from build123d import *

# Parameters (mm, degrees)
BOSS_EXTRUDE1_DEPTH = 10.7
BOSS_EXTRUDE2_DEPTH = 2
CUT_EXTRUDE2_DEPTH  = 17.842989329
CHAMFER1_SIZE       = 0.4


with BuildPart() as part:
    # Sketch1 → Boss-Extrude1 (new body)
    with BuildSketch(Plane.XY):
        Polygon((0, -6.142777017), (2.175697935, -3.768419365), (5.319800946, -3.071388508), (4.351395869, 0), (5.319800946, 3.071388508), (2.175697935, 3.768419365), (0, 6.142777017), (-2.175697935, 3.768419365), (-5.319800946, 3.071388508), (-4.351395869, 0), (-5.319800946, -3.071388508), (-2.175697935, -3.768419365), align=None)
    extrude(amount=-BOSS_EXTRUDE1_DEPTH)

    # Sketch2 → Boss-Extrude2 (add)
    # profile 1 of 2: a face of its own
    with BuildSketch(Plane.XY):
        Polygon((5.924189557, 0), (7.242620565, 4.181528933), (2.962094779, 5.130498653), (0, 8.363057866), (-2.962094779, 5.130498653), (-7.242620565, 4.181528933), (-5.924189557, 0), (-7.242620565, -4.181528933), (-2.962094779, -5.130498653), (0, -8.363057866), (2.962094779, -5.130498653), (7.242620565, -4.181528933), align=None)
        Polygon((5.319800946, -3.071388508), (4.351395869, 0), (5.319800946, 3.071388508), (2.175697935, 3.768419365), (0, 6.142777017), (-2.175697935, 3.768419365), (-5.319800946, 3.071388508), (-4.351395869, 0), (-5.319800946, -3.071388508), (-2.175697935, -3.768419365), (0, -6.142777017), (2.175697935, -3.768419365), align=None, mode=Mode.SUBTRACT)
    # profile 2 of 2: a face of its own
    with BuildSketch(Plane.XY):
        Polygon((2.175697935, -3.768419365), (5.319800946, -3.071388508), (4.351395869, 0), (5.319800946, 3.071388508), (2.175697935, 3.768419365), (0, 6.142777017), (-2.175697935, 3.768419365), (-5.319800946, 3.071388508), (-4.351395869, 0), (-5.319800946, -3.071388508), (-2.175697935, -3.768419365), (0, -6.142777017), align=None)
    extrude(amount=BOSS_EXTRUDE2_DEPTH)

    # Sketch3 → Cut-Extrude2 (cut, through all)
    with BuildSketch(Plane.XY.offset(2)):
        with BuildLine():
            ThreePointArc((1.65, 0), (1.442792528, 0.800530899), (0.87321246, 1.4))
            Line((0.87321246, 1.4), (-0.87321246, 1.4))
            ThreePointArc((-0.87321246, 1.4), (-1.442792528, 0.800530899), (-1.65, 0))
            ThreePointArc((-1.65, 0), (0, -1.65), (1.65, 0))
        make_face()
    extrude(amount=-CUT_EXTRUDE2_DEPTH, mode=Mode.SUBTRACT)

    # Chamfer1
    chamfer1_edges = [part.edges().sort_by_distance(p)[0] for p in [
        (3.74774944, -3.419903937, 0),
        (1.087848967, -4.955598191, 0),
        (-1.087848967, -4.955598191, 0),
        (-3.74774944, -3.419903937, 0),
        (-4.835598408, -1.535694254, 0),
        (-4.835598408, 1.535694254, 0),
        (-3.74774944, 3.419903937, 0),
        (-1.087848967, 4.955598191, 0),
        (1.087848967, 4.955598191, 0),
        (3.74774944, 3.419903937, 0),
        (4.835598408, 1.535694254, 0),
        (4.835598408, -1.535694254, 0),
    ]]
    chamfer(chamfer1_edges, length=CHAMFER1_SIZE)


solid = part.part
The listing builds one solid part. Answer for the finished solid, in the listing's coordinates (mm). A direction names the side the tool comes from. Give positions to 0.01 mm unless a question says otherwise; leave off trailing zeros. Loops run counter-clockwise (first coordinate to the right, second up) from the corner with the lowest first, then second, coordinate; pieces in that order, holes last. Notation, with made-up numbers: (26, 11) - (63, 11) arc R23 cw to (63, 21) - close; hole circle Ø1 at (8, 27.25). An arc over 180 degrees is marked (long way). Write each question's results on one line, items separated by ' | '.
1. For a pull along Y with two mould halves and no side action, classify faces 1 (the face through (1.1, 1.5, -10.7)), 2 (the face through (3.77, 3.415, -5.478)), 3 (the face through (3.726, -3.425, -5.478)), 4 (the face through (-4.829, -1.514, -5.478)) as +Y half, -Y half, draft (parallel to the pull), parting line (faces both ways), or undercut.
Resolved:
face 1: draft | face 2: +Y half | face 3: -Y half | face 4: undercut
2. Find section B-B, the plane y = 0.5. Write down the section's boundary in (x, z), then the cut area to 3 significant figures.
Resolved:
outline: (-6.08, 0) - (-4.93, 0) - (-4.51, -0.4) - (-4.51, -10.7) - (-1.57, -10.7) - (-1.57, 2) - (-6.08, 2) - close; (1.57, -10.7) - (4.51, -10.7) - (4.51, -0.4) - (4.93, 0) - (6.08, 0) - (6.08, 2) - (1.57, 2) - close | area: 81.0 mm^2
3. Which of the six approach directions +Z, -Z, +X, -X, +Y, -Y give full straight-line access (tool end or side, diameter ignored) to faces 5 (the face through (5.1, 1.7, -0.2)), 6 (the face through (-1.103, -5.231, -0.203)), 7 (the face through (-1.07, 5.27, -0.2)), 8 (the face through (-5.1, 1.7, -0.2)), 9 (the face through (0, 1.4, -4))?
Resolved:
face 5: -Z, +X | face 6: -Z, -X, -Y | face 7: -Z, -X, +Y | face 8: -Z, -X | face 9: +Z, -Z
4. Consider probe 1 along Y at (x, z) = (0.75, -10); probe 2 along Y at (x, z) = (-1.5, -2.25); probe 3 along Z at (x, y) = (-6, -0.75). Determine where each line is inside the solid, lowest interval first. Write a range as from..to.
Resolved:
probe 1: y = -5.32..-1.47, 1.4..5.32 | probe 2: y = -4.51..-0.69, 0.69..4.51 | probe 3: z = 0..2
5. Find section D-D, the plane x = 0.5. Write down the section's boundary in (y, z), then the cut area to 3 significant figures.
Resolved:
outline: (-7.82, 0) - (-6.19, 0) - (-5.6, -0.4) - (-5.6, -10.7) - (-1.57, -10.7) - (-1.57, 2) - (-7.82, 2) - close; (1.4, -10.7) - (5.6, -10.7) - (5.6, -0.4) - (6.19, 0) - (7.82, 0) - (7.82, 2) - (1.4, 2) - close | area: 114 mm^2
6. Flat-ended cylindrical pins translate along their axes: P1, Ø4, axis at x = 4, z = -2.5, coming from the -Y side; P2, Ø2, axis at y = 5, z = -2, coming from the -X side; P3, Ø0.9, axis at x = -0.5, z = -5, coming from the -Y side. Find the tip coordinate at first contact, or state that the pin passes through.
Resolved:
P1: stops at y = -3.96 | P2: stops at x = -1.96 | P3: stops at y = -6.09
7. Find section A-A, the plane z = -9.25. Write down the section's boundary in (x, y), then the cut area to 3 significant figures.
Resolved:
outline: (-5.32, -3.07) - (-2.18, -3.77) - (0, -6.14) - (2.18, -3.77) - (5.32, -3.07) - (4.35, 0) - (5.32, 3.07) - (2.18, 3.77) - (0, 6.14) - (-2.18, 3.77) - (-5.32, 3.07) - (-4.35, 0) - close; hole (-0.87, 1.4) arc R1.65 ccw (long way) to (0.87, 1.4) - close | area: 71.9 mm^2
8. Find section C-C, the plane x = 4. Write down the section's boundary in (y, z), then the cut area to 3 significant figures.
Resolved:
outline: (-4.9, 0) - (-3.77, 0) - (-3.36, -0.4) - (-3.36, -10.7) - (3.36, -10.7) - (3.36, -0.4) - (3.77, 0) - (4.9, 0) - (4.9, 2) - (-4.9, 2) - close | area: 91.8 mm^2
